Part model, mm, in its own coordinate system. Face numbers are marked on the shaded views. A direction names the side the tool comes from. Coordinates: 2 decimals unless noted, no trailing zeros. Order: outer loops, then holes, each group sorted by start corner. A loop starts at its lowest first (then second) coordinate and runs counter-clockwise, first axis right, second up. Notation, with made-up numbers: (40, 71) - (74, 71) arc R33 ccw to (74, 109) - close; hole circle Ø7 at (-11.75, 40). An arc over 180 degrees is marked (long way). Use a Markdown table: item, result. Add a question column.
1) Saw through at A-A on x = 0. List the corners of the cut face in (y, z).
2) Two-plate mould, pull along X, no slides. Class the marked faces 3, 4 and 5: +X half, -X half, draft (parallel to the pull), parting line (faces both ways), or undercut.
3) Drop flat-ended pins along their axis: P1, Ø6, axis at y = -36.5, z = 8, coming from the +X side; P2, Ø18, axis at x = 0, y = -100, coming from the -Z side; P3, Ø1, axis at y = 1.5, z = 4.5, coming from the -X side; P4, Ø1.5, axis at x = 9, z = 9, coming from the +Y side. Give the stop position or say it passes through.
4) Saw through at C-C on z = -1. List the corners of the cut face in (x, y), then the cut area to 3 significant figures.
5) Tool access for the marked faces 1 and 2: list every direction of +Z, -Z, +X, -X, +Y, -Y with a clear straight run to the whole face (end or side of a thin tool).
6) Saw through at B-B on y = 0. List the corners of the cut face in (x, z), then the cut area to 3 significant figures.
7) Wall check: L1, parallel to Y at x = 0, z = 6.25; L2, parallel to Y at x = -2.5, z = -7.75; L3, parallel to X at y = -24.5, z = 6.5. Give the ranges that are in metal, low to high. Write a range as [from, to].
```python
from build123d import *

# Parameters (mm, degrees)
SKETCH1_R               = 25
SKETCH1_R_2             = 15
BOSS_EXTRUDE1_DEPTH     = 12.5
SKETCH2_W               = 30
SKETCH2_H               = 20
BOSS_EXTRUDE2_DEPTH     = 100
SKETCH3_R               = 25
SKETCH3_R_2             = 15
BOSS_EXTRUDE3_DEPTH     = 12.5
CUT_EXTRUDE1_DEPTH      = 129.086884574
CUT_EXTRUDE1_DEPTH_BACK = 129.086884574
SKETCH4_R               = 15


with BuildPart() as part:
    # Sketch1 → Boss-Extrude1 (new, symmetric)
    with BuildSketch(Plane.XY):
        Circle(SKETCH1_R)
        Circle(SKETCH1_R_2, mode=Mode.SUBTRACT)
    extrude(amount=BOSS_EXTRUDE1_DEPTH, both=True)

    # Sketch2 → Boss-Extrude2 (add)
    with BuildSketch(Plane(origin=(0, 0, 0), x_dir=(1, 0, 0), z_dir=(0, 1, 0))):
        Rectangle(SKETCH2_W, SKETCH2_H)
    extrude(amount=-BOSS_EXTRUDE2_DEPTH)

    # Sketch3 → Boss-Extrude3 (add, symmetric)
    with BuildSketch(Plane.XY):
        with Locations((0, -100)):
            Circle(SKETCH3_R)
        with Locations((0, -100)):
            Circle(SKETCH3_R_2, mode=Mode.SUBTRACT)
    extrude(amount=BOSS_EXTRUDE3_DEPTH, both=True)

    # Sketch4 → Cut-Extrude1 (cut, two sides: drawn at the far end of the back side and taken through both)
    with BuildSketch(Plane.XY.offset(-CUT_EXTRUDE1_DEPTH_BACK)):
        Circle(SKETCH4_R)
        with Locations((0, -100)):
            Circle(SKETCH4_R)
    extrude(amount=CUT_EXTRUDE1_DEPTH + CUT_EXTRUDE1_DEPTH_BACK, mode=Mode.SUBTRACT)


solid = part.part
```
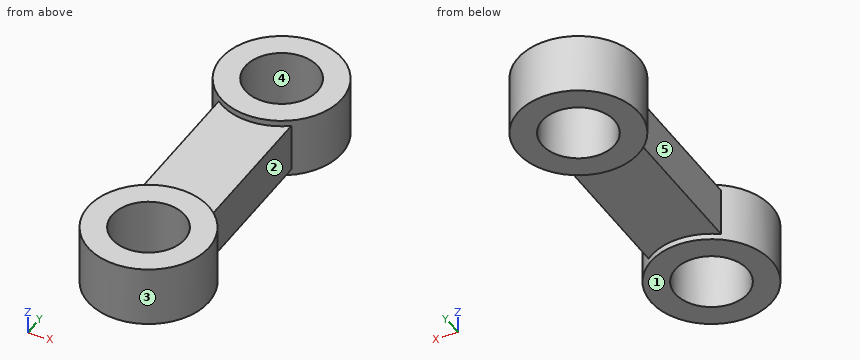
Results are:
| question | item | result |
|---|---|---|
| 1 | outline | (-125, -12.5) - (-115, -12.5) - (-115, 12.5) - (-125, 12.5) - close; (-85, -12.5) - (-75, -12.5) - (-75, -10) - (-25, -10) - (-25, -12.5) - (-15, -12.5) - (-15, 12.5) - (-25, 12.5) - (-25, 10) - (-75, 10) - (-75, 12.5) - (-85, 12.5) - close; (15, -12.5) - (25, -12.5) - (25, 12.5) - (15, 12.5) - close |
| 2 | face 3 | parting line |
| 2 | face 4 | undercut |
| 2 | face 5 | -X half |
| 3 | P1 | x = 15 |
| 3 | P2 | through |
| 3 | P3 | x = -24.98 |
| 3 | P4 | y = 23.6 |
| 4 | outline | (-15, -80) arc R25 ccw (long way) to (15, -80) - (15, -20) arc R25 ccw (long way) to (-15, -20) - close; hole circle Ø30 at (0, -100); hole circle Ø30 at (0, 0) |
| 4 | area | 4,110 mm2 |
| 5 | face 1 | -Z, +X, -X, +Y, -Y |
| 5 | face 2 | +Z, -Z, +X |
| 6 | outline | (-25, -12.5) - (-15, -12.5) - (-15, 12.5) - (-25, 12.5) - close; (15, -12.5) - (25, -12.5) - (25, 12.5) - (15, 12.5) - close |
| 6 | area | 500 mm2 |
| 7 | L1 | [-125, -115], [-85, -15], [15, 25] |
| 7 | L2 | [-124.87, -114.79], [-85.21, -14.79], [14.79, 24.87] |
| 7 | L3 | [-15, 15] |
